Verification items for this drawing (mm, ordinates from the low corner). A direction names the side the tool comes from. Give positions to 0.01 mm unless a question says otherwise; leave off trailing zeros. Loops run counter-clockwise (first coordinate to the right, second up) from the corner with the lowest first, then second, coordinate; pieces in that order, holes last. Notation, with made-up numbers: M -23.75,50 L -3.75,50 A17 ccw -3.75,75 Z; hole C 31,84 d11. An arc over 180 degrees is marked long. Answer in a Markdown table with one row per item.
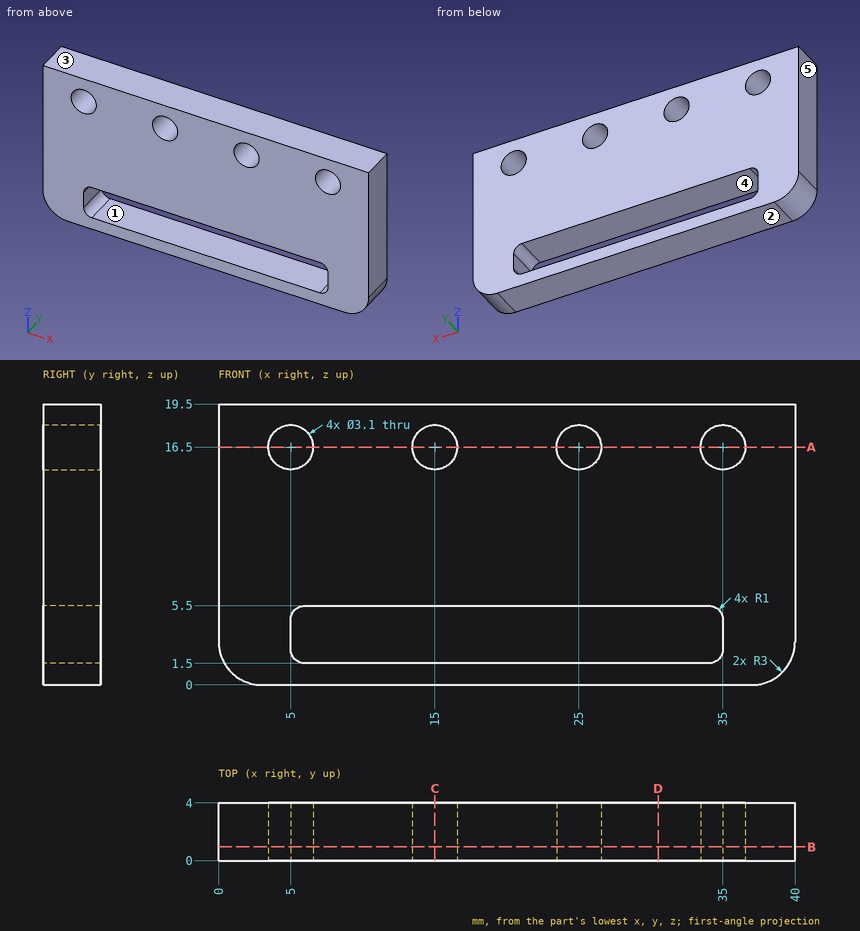
Item 1: Sectioned sample at C-C (x = 15). Record the cut outline in (y, z).
Reported:
| item | result |
|---|---|
| outline | M 0,0 L 4,0 L 4,1.5 L 0,1.5 Z; M 0,5.5 L 4,5.5 L 4,14.95 L 0,14.95 Z; M 0,18.05 L 4,18.05 L 4,19.5 L 0,19.5 Z |
Item 2: Sectioned sample at D-D (x = 30.5). Record the cut outline in (y, z), and give its area (3 significant figures).
Reported:
| item | result |
|---|---|
| outline | M 0,0 L 4,0 L 4,1.5 L 0,1.5 Z; M 0,5.5 L 4,5.5 L 4,19.5 L 0,19.5 Z |
| area | 62.0 mm^2 |
Item 3: Sectioned sample at A-A (z = 16.5). Record the cut outline in (x, y), and give its area (3 significant figures).
Reported:
| item | result |
|---|---|
| outline | M 0,0 L 3.45,0 L 3.45,4 L 0,4 Z; M 6.55,0 L 13.45,0 L 13.45,4 L 6.55,4 Z; M 16.55,0 L 23.45,0 L 23.45,4 L 16.55,4 Z; M 26.55,0 L 33.45,0 L 33.45,4 L 26.55,4 Z; M 36.55,0 L 40,0 L 40,4 L 36.55,4 Z |
| area | 110 mm^2 |
Item 4: Sectioned sample at B-B (y = 0.95). Record the cut outline in (x, z).
Reported:
| item | result |
|---|---|
| outline | M 0,3 A3 ccw 3,0 L 37,0 A3 ccw 40,3 L 40,19.5 L 0,19.5 Z; hole C 5,16.5 d3.1; hole M 5,2.5 A1 ccw 6,1.5 L 34,1.5 A1 ccw 35,2.5 L 35,4.5 A1 ccw 34,5.5 L 6,5.5 A1 ccw 5,4.5 Z; hole C 15,16.5 d3.1; hole C 25,16.5 d3.1; hole C 35,16.5 d3.1 |
Item 5: Scan lines: L1, parallel to Z at x = 25, y = 1.2; L2, parallel to X at y = 2.6, z = 16.5; L3, parallel to X at y = 2.2, z = 15.5. Record each from-to range of solid material in increasing order. Write a range as [from, to].
Reported:
| item | result |
|---|---|
| L1 | z = [0, 1.5], [5.5, 14.95], [18.05, 19.5] |
| L2 | x = [0, 3.45], [6.55, 13.45], [16.55, 23.45], [26.55, 33.45], [36.55, 40] |
| L3 | x = [0, 3.82], [6.18, 13.82], [16.18, 23.82], [26.18, 33.82], [36.18, 40] |
Item 6: Tool access check on the marked faces 4 and 5. Record the directions out of +Z, -Z, +X, -X, +Y, -Y that give a thin tool (end or side, any length) a straight path to the whole face; none if there is none.
Reported:
| item | result |
|---|---|
| face 4 | +Y, -Y |
| face 5 | +Z, -Z, -X, +Y, -Y |
Item 7: Release check for a two-part mould opening along Z. For the marked faces 1, 2 and 3 record: released by +Z, released by -Z, zero draft, split by the parting line, or undercut.
Reported:
| item | result |
|---|---|
| face 1 | undercut |
| face 2 | released by -Z |
| face 3 | released by +Z |
Item 8: Go/stop test with a flat-tipped pin: pin 1 (3 mm diameter, centred on x = 35, z = 16.5, fed in from -Y). Record where the tip stops, or that it passes through.
Reported:
| item | result |
|---|---|
| pin 1 | passes through |
